Here's how the part is built. I have some questions about the finished solid (model axes, mm). Round coordinates to 2 decimals unless told otherwise and drop trailing zeros. Order: outer loops, then holes, each group sorted by start corner. A loop starts at its lowest first (then second) coordinate and runs counter-clockwise, first axis right, second up. Notation, with made-up numbers: M 3,26.25 L 62,26.25 A24 cw 62,47.25 Z; hole C 69.5,5 d4. An arc over 180 degrees is marked long. Answer as CSV lines item,"result". Start each with the question number.
Autodesk Inventor part; units mm, degrees
ref_plane "YZ Plane" through (0, 0, 0) normal (1, 0, 0) x (0, 1, 0)
ref_plane "XZ Plane" through (0, 0, 0) normal (0, 1, 0) x (-1, 0, 0)
ref_plane "XY Plane" through (0, 0, 0) normal (0, 0, 1) x (1, 0, 0)
sketch "Sketch1" plane through (0, 0, 0) normal (0, 1, 0) x (-1, 0, 0)
  line L0 (0, 0) -> (-590, 0)
  line L1 (-590, 0) -> (-590, -165.9671)
  line L2 (-590, -165.9671) -> (0, -165.9671)
  line L3 (0, -165.9671) -> (0, 0)
  line L4 (0, -165.9671) -> (0, -270)
  line L5 (0, -270) -> (-590, -165.9671)
  dimension "d0" = 590
  dimension "d28" = 270
  dimension "d29" = 10
extrude "Extrusion1" add sketch "Sketch1" along normal blind 3
sketch "Sketch3" plane through (0, 3, 0) normal (0, 1, 0) x (1, 0, 0)
  circle A0 centre (585.75, 41.75) radius 1.25
  circle A1 centre (585.75, 78.75) radius 1.25
  line L0 (590, 0) -> (590, 165.9671)
  line L1 (0, 0) -> (590, 0)
  dimension "d15" = 2.5
  dimension "d16" = 4.25
  dimension "d17" = 4.25
  dimension "d18" = 2.5
  dimension "d19" = 41.75
  dimension "d20" = 37
extrude "Extrusion3" cut sketch "Sketch3" along normal through all both and the other way through all
sketch "Sketch4" plane through (0, 3, 0) normal (0, 1, 0) x (1, 0, 0)
  circle A0 centre (490, 60) radius 12
  line L0 (0, 0) -> (590, 0)
  line L1 (590, 0) -> (590, 165.9671)
  dimension "d23" = 24
  dimension "d24" = 60
  dimension "d25" = 100
extrude "Extrusion4" cut sketch "Sketch4" against normal through all
equation "\"d16\" = d17"
equation "\"d18\" = d15"
properties part number "pinball-case-left-wall-outer"
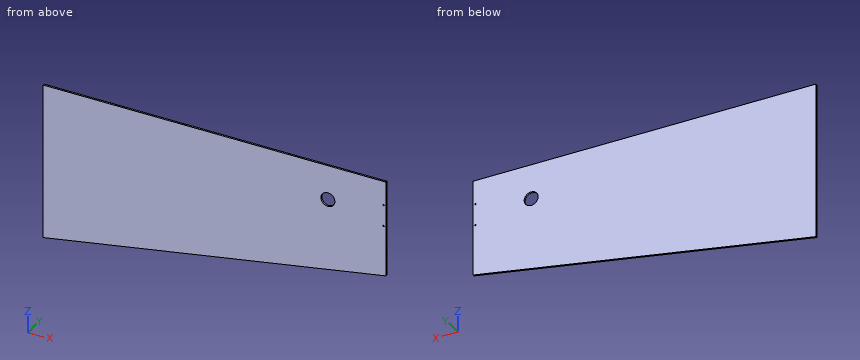
Item 1: If we section it at D-D on z = -223.5: Please give me the cut outline in (x, y), and give its area (3 significant figures).
Item 2: If we section it at B-B on z = -60: Please give me the cut outline in (x, y), and give its area (3 significant figures).
Item 3: If we section it at A-A on y = 1.9: Please give me the cut outline in (x, z).
Item 4: If we section it at C-C on x = 490: Please give me the cut outline in (y, z).
Item 5: If I drill on line 1 along X through (y, z) = (1.9, -41.75); line 2 along Z through (x, y) = (585.75, 1.8); line 3 along Z through (x, y) = (490, 1.3), over which ranges is the centre line in solid material (lowest first)?
Geometry says:
1,outline,"M 0,0 L 263.71,0 L 263.71,3 L 0,3 Z"
1,area,"791 mm²"
2,outline,"M 0,0 L 478,0 L 478,3 L 0,3 Z; M 502,0 L 590,0 L 590,3 L 502,3 Z"
2,area,"1,700 mm²"
3,outline,"M 0,-270 L 590,-165.97 L 590,0 L 0,0 Z; hole C 490,-60 d24; hole C 585.75,-78.75 d2.5; hole C 585.75,-41.75 d2.5"
4,outline,"M 0,-183.6 L 3,-183.6 L 3,-72 L 0,-72 Z; M 0,-48 L 3,-48 L 3,0 L 0,0 Z"
5,line 1,"0 to 584.5, 587 to 590"
5,line 2,"-166.72 to -80, -77.5 to -43, -40.5 to 0"
5,line 3,"-183.6 to -72, -48 to 0"
